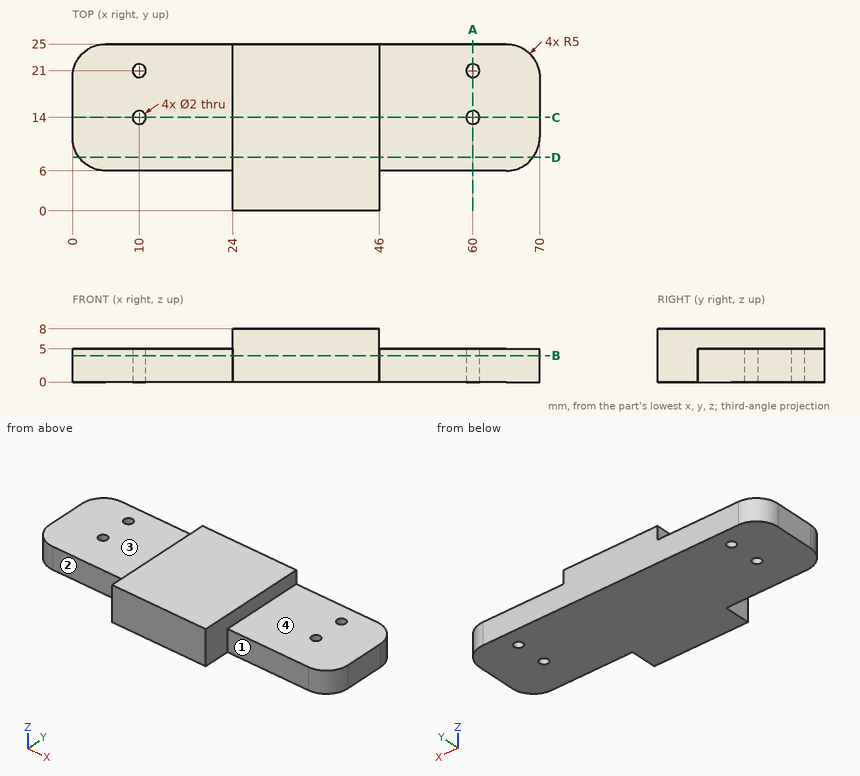
Geometry check sheet. Reference: drawing and pictorial views, mm from the part's lowest x, y, z. A direction names the side the tool comes from. Give positions to 0.01 mm unless a question says otherwise; leave off trailing zeros. Order: outer loops, then holes, each group sorted by start corner. A loop starts at its lowest first (then second) coordinate and runs counter-clockwise, first axis right, second up. Notation, with made-up numbers: M 39,60 L 68,60 A24 ccw 68,90 Z; hole C 78.25,78 d6. An arc over 180 degrees is marked long. Answer in a Markdown table with one row per item. Add a question column.
Q1. Sectioned sample at C-C, the plane y = 14. Record the boundary of the cut face in (x, z), and give its area (3 significant figures).
Q2. Sectioned sample at A-A, the plane x = 60. Record the boundary of the cut face in (y, z).
Q3. Thickness scan on L1, parallel to Y at x = 60, z = 2.8; L2, parallel to Y at x = 23, z = 0.5; L3, parallel to X at y = 21, z = 6. Record the ranges inside material, lowest first.
Q4. Gauge pin test, flat ends, axial feed: pin 1 Ø15 at (x, y) = (63.5, 11) entering from +Z; pin 2 Ø1.6 at (x, y) = (10, 21) entering from +Z; pin 3 Ø2.5 at (x, z) = (19, 1.5) entering from -Y. Record the tip position at first contact, or that the pin passes through.
Q5. Access from +Z, -Z, +X, -X, +Y, -Y to the whole of each face (thin tool, end or side, straight path). Record for the marked faces 1, 2, 3 and 4.
Q6. Sectioned sample at D-D, the plane y = 8. Record the boundary of the cut face in (x, z).
Q7. Sectioned sample at B-B, the plane z = 4. Record the boundary of the cut face in (x, y).
Verdict:
| question | item | result |
|---|---|---|
| 1 | outline | M 0,0 L 9,0 L 9,5 L 0,5 Z; M 11,0 L 59,0 L 59,5 L 46,5 L 46,8 L 24,8 L 24,5 L 11,5 Z; M 61,0 L 70,0 L 70,5 L 61,5 Z |
| 1 | area | 396 mm² |
| 2 | outline | M 6,0 L 13,0 L 13,5 L 6,5 Z; M 15,0 L 20,0 L 20,5 L 15,5 Z; M 22,0 L 25,0 L 25,5 L 22,5 Z |
| 3 | L1 | 6 to 13, 15 to 20, 22 to 25 |
| 3 | L2 | 6 to 25 |
| 3 | L3 | 24 to 46 |
| 4 | pin 1 | z = 5 |
| 4 | pin 2 | through |
| 4 | pin 3 | y = 6 |
| 5 | face 1 | +Z, -Z, +X, -Y |
| 5 | face 2 | +Z, -Z, -X, -Y |
| 5 | face 3 | +Z, -X, +Y, -Y |
| 5 | face 4 | +Z, +X, +Y, -Y |
| 6 | outline | M 1,0 L 69,0 L 69,5 L 46,5 L 46,8 L 24,8 L 24,5 L 1,5 Z |
| 7 | outline | M 0,11 A5 ccw 5,6 L 24,6 L 24,0 L 46,0 L 46,6 L 65,6 A5 ccw 70,11 L 70,20 A5 ccw 65,25 L 5,25 A5 ccw 0,20 Z; hole C 10,14 d2; hole C 10,21 d2; hole C 60,14 d2; hole C 60,21 d2 |
